```python
from build123d import *

# Parameters (mm, degrees)
F0_W     = 6
F0_H     = 5
F0_W_2   = 30
F1_DEPTH = 2


with BuildPart() as f1:
    # F0 (on Top) → F1 (new body)
    with BuildSketch(Plane.XY):
        with BuildLine():
            ThreePointArc((-45, -1.5), (-46.5, 0), (-45, 1.5))
            Line((-45, 1.5), (-45, 5))
            ThreePointArc((-45, 5), (-50, 0), (-45, -5))
            Line((-45, -5), (-45, -1.5))
        make_face()
        with BuildLine():
            ThreePointArc((-45, 5), (-42.576157338, 4.3732124062), (-40.76000848, 2.6499947))
            Line((-40.76000848, 2.6499947), (-21, 15))
            Line((-21, 15), (-21, 20))
            Line((-21, 20), (-45, 5))
        make_face()
        with BuildLine():
            Line((-21, -15), (-40.76000848, -2.6499947))
            ThreePointArc((-40.76000848, -2.6499947), (-42.576157338, -4.3732124062), (-45, -5))
            Line((-45, -5), (-21, -20))
            Line((-21, -20), (-21, -15))
        make_face()
        with BuildLine():
            ThreePointArc((50, 0), (48.5355339059, 3.5355339059), (45, 5))
            Line((45, 5), (45, 1.5))
            ThreePointArc((45, 1.5), (46.0606601718, 1.0606601718), (46.5, 0))
            ThreePointArc((46.5, 0), (46.0606601718, -1.0606601718), (45, -1.5))
            Line((45, -1.5), (45, -5))
            ThreePointArc((45, -5), (48.5355339059, -3.5355339059), (50, 0))
        make_face()
        with BuildLine():
            Line((21, 20), (21, 15))
            Line((21, 15), (40.76000848, 2.6499947))
            ThreePointArc((40.76000848, 2.6499947), (42.576157338, 4.3732124062), (45, 5))
            Line((45, 5), (21, 20))
        make_face()
        with BuildLine():
            Line((40.76000848, -2.6499947), (21, -15))
            Line((21, -15), (21, -20))
            Line((21, -20), (45, -5))
            ThreePointArc((45, -5), (42.576157338, -4.3732124062), (40.76000848, -2.6499947))
        make_face()
        with Locations((-18, 17.5)):
            Rectangle(F0_W, F0_H)
        with Locations((0, 17.5)):
            Rectangle(F0_W_2, F0_H)
        with Locations((18, 17.5)):
            Rectangle(F0_W, F0_H)
        with BuildLine():
            ThreePointArc((-45, 1.5), (-44.2728472014, 1.3119637219), (-43.728002544, 0.79499841))
            Line((-43.728002544, 0.79499841), (-40.76000848, 2.6499947))
            ThreePointArc((-40.76000848, 2.6499947), (-42.576157338, 4.3732124062), (-45, 5))
            Line((-45, 5), (-45, 1.5))
        make_face()
        with BuildLine():
            Line((-40.76000848, -2.6499947), (-43.728002544, -0.79499841))
            ThreePointArc((-43.728002544, -0.79499841), (-44.2728472014, -1.3119637219), (-45, -1.5))
            Line((-45, -1.5), (-45, -5))
            ThreePointArc((-45, -5), (-42.576157338, -4.3732124062), (-40.76000848, -2.6499947))
        make_face()
        with BuildLine():
            ThreePointArc((45, 5), (42.576157338, 4.3732124062), (40.76000848, 2.6499947))
            Line((40.76000848, 2.6499947), (43.728002544, 0.79499841))
            ThreePointArc((43.728002544, 0.79499841), (44.2728472014, 1.3119637219), (45, 1.5))
            Line((45, 1.5), (45, 5))
        make_face()
        with BuildLine():
            Line((43.728002544, -0.79499841), (40.76000848, -2.6499947))
            ThreePointArc((40.76000848, -2.6499947), (42.576157338, -4.3732124062), (45, -5))
            Line((45, -5), (45, -1.5))
            ThreePointArc((45, -1.5), (44.2728472014, -1.3119637219), (43.728002544, -0.79499841))
        make_face()
        with Locations((-18, -17.5)):
            Rectangle(F0_W, F0_H)
        with Locations((18, -17.5)):
            Rectangle(F0_W, F0_H)
        with BuildLine():
            ThreePointArc((-43.728002544, 0.79499841), (-43.5581268808, 0.4135237696), (-43.5, 0))
            Line((-43.5, 0), (-40, 0))
            ThreePointArc((-40, 0), (-40.1937562692, 1.3784125652), (-40.76000848, 2.6499947))
            Line((-40.76000848, 2.6499947), (-43.728002544, 0.79499841))
        make_face()
        with BuildLine():
            Line((-40, 0), (-43.5, 0))
            ThreePointArc((-43.5, 0), (-43.5581268808, -0.4135237696), (-43.728002544, -0.79499841))
            Line((-43.728002544, -0.79499841), (-40.76000848, -2.6499947))
            ThreePointArc((-40.76000848, -2.6499947), (-40.1937562692, -1.3784125652), (-40, 0))
        make_face()
        with BuildLine():
            ThreePointArc((40.76000848, 2.6499947), (40.1937562692, 1.3784125652), (40, 0))
            Line((40, 0), (43.5, 0))
            ThreePointArc((43.5, 0), (43.5581268808, 0.4135237696), (43.728002544, 0.79499841))
            Line((43.728002544, 0.79499841), (40.76000848, 2.6499947))
        make_face()
        with BuildLine():
            Line((43.5, 0), (40, 0))
            ThreePointArc((40, 0), (40.1937562692, -1.3784125652), (40.76000848, -2.6499947))
            Line((40.76000848, -2.6499947), (43.728002544, -0.79499841))
            ThreePointArc((43.728002544, -0.79499841), (43.5581268808, -0.4135237696), (43.5, 0))
        make_face()
        Polygon((-21, 15), (-21, 0), (21, 0), (21, 15), (15, 15), (-15, 15), align=None)
        Polygon((21, 0), (-21, 0), (-21, -15), (-15, -15), (15, -15), (21, -15), align=None)
        with Locations((0, -17.5)):
            Rectangle(F0_W_2, F0_H)
    extrude(amount=F1_DEPTH)


solid = f1.part
```
CAD build for the part. Positions are in the model's coordinates, mm. A direction names the side the tool comes from. Round coordinates to 2 decimals unless told otherwise and drop trailing zeros. Order: outer loops, then holes, each group sorted by start corner. A loop starts at its lowest first (then second) coordinate and runs counter-clockwise, first axis right, second up. Notation, with made-up numbers: (-27, -34.5) - (21, -34.5) arc R22 ccw to (21, -28.5) - close; hole circle Ø5 at (64.5, 18.5). An arc over 180 degrees is marked (long way). Answer as CSV lines item,"result". Start each with the question number.
1. Pin check, flat tip, straight feed: pin 1 (0.6 mm diameter, centred on y = -4, z = 1.5, fed in from -X). Stop position of the tip, or through.
2. Tool access for faces 1 (the face through (31.018, -8.739, 0.986)), 2 (the face through (-50, 0, 1)): list every direction of +Z, -Z, +X, -X, +Y, -Y with a clear straight run to the whole face (end or side of a thin tool).
3. Saw through at A-A, the plane y = 9.5. Write the cut outline in (x, z), and give its area (3 significant figures).
4. Saw through at C-C, the plane x = -24. Write the cut outline in (y, z) (3 decimals).
5. Pull direction Y, two halves, no side cores. Call faces 3 (the face through (-33.168, -12.395, 0.986)), 4 (the face through (-31.018, 8.739, 0.986)), 5 (the face through (-32.832, 12.605, 0.986)), 6 (the face through (21, 0, 1)): +Y half, -Y half, draft (parallel to the pull), parting line (faces both ways), or undercut.
6. Saw through at B-B, the plane z = 0.35. Write the cut outline in (x, y) (3 decimals).
7. Drill centre lines: L1, parallel to X at y = 11.5, z = 1.35; L2, parallel to X at y = -10.5, z = 1.05; L3, parallel to Y at x = -26, z = 1.85 (3 decimals). Where is each one in solid material? Low to high. Write a range as [from, to].
Model answer:
1,pin 1,"stops at x = -48.36"
2,face 1,"+Z, -Z"
2,face 2,"+Z, -Z, -X"
3,outline,"(-37.8, 0) - (-29.8, 0) - (-29.8, 2) - (-37.8, 2) - close; (-21, 0) - (21, 0) - (21, 2) - (-21, 2) - close; (29.8, 0) - (37.8, 0) - (37.8, 2) - (29.8, 2) - close"
3,area,"116 mm²"
4,outline,"(-18.125, 0) - (-13.125, 0) - (-13.125, 2) - (-18.125, 2) - close; (13.125, 0) - (18.125, 0) - (18.125, 2) - (13.125, 2) - close"
5,face 3,"-Y half"
5,face 4,"undercut"
5,face 5,"+Y half"
5,face 6,"undercut"
6,outline,"(-45, -5) - (-21, -20) - (21, -20) - (45, -5) arc R5 ccw to (45, 5) - (21, 20) - (-21, 20) - (-45, 5) arc R5 ccw to start; hole circle Ø3 at (-45, 0); hole (-40.76, -2.65) - (-21, -15) - (-21, 15) - (-40.76, 2.65) arc R5 cw to start; hole (21, -15) - (40.76, -2.65) arc R5 cw to (40.76, 2.65) - (21, 15) - close; hole circle Ø3 at (45, 0)"
7,L1,"x = [-34.6, -26.6], [-21, 21], [26.6, 34.6]"
7,L2,"x = [-36.2, -28.2], [-21, 21], [28.2, 36.2]"
7,L3,"y = [-16.875, -11.875], [11.875, 16.875]"
